from build123d import *

# Parameters (mm, degrees)
F1_DEPTH = 25
F2_R     = 2.5
F3_DEPTH = 15


with BuildPart() as f1:
    # F0 (on Front) → F1 (new body)
    with BuildSketch(Plane.XZ):
        Polygon((3.64, 10), (0, 0), (20, 0), (16.36, 10), (10, 10), align=None)
    extrude(amount=F1_DEPTH)

    # F2 (on Top) → F3 (join)
    with BuildSketch(Plane.XY):
        with Locations((10, -12.5)):
            Circle(F2_R)
    extrude(amount=F3_DEPTH)


solid = f1.part
Here's how the part is built. I have some questions about the finished solid (model axes, mm). A direction names the side the tool comes from. Give positions to 0.01 mm unless a question says otherwise; leave off trailing zeros. Order: outer loops, then holes, each group sorted by start corner. A loop starts at its lowest first (then second) coordinate and runs counter-clockwise, first axis right, second up. Notation, with made-up numbers: M -15,-3 L 29,-3 A22 ccw 29,9 Z; hole C -22,-11 d2. An arc over 180 degrees is marked long. Answer as a JSON object with one key per item and string values. Group by question number.
1) Suppose I cut it at B-B, the plane x = 10. Write out the boundary of the cut face in (y, z), plus the area to 3 significant figures.
2) Suppose I cut it at A-A, the plane y = -12.5. Write out the boundary of the cut face in (x, z), plus the area to 3 significant figures.
3) On a 3-axis mill with a long thin cutter (end or side, diameter ignored), from which of +Z, -Z, +X, -X, +Y, -Y can I reach the whole of each face in a straight line? I mean faces 1 (the flat face through (10, 0, 5)), 2 (the cylindrical face through (9.46, -14.94, 12.46)). Say none if no direction works.
4) Please list where these lines run through material, in increasing order: L1, parallel to Z at x = 7.5, y = -6; L2, parallel to Y at x = 11.25, z = 11.5; L3, parallel to X at y = -4.25, z = 6.75. Write a range as [from, to].
5) Suppose I cut it at C-C, the plane z = 12.5. Write out the boundary of the cut face in (x, y).
6) Suppose I cut it at D-D, the plane y = -5. Write out the boundary of the cut face in (x, z).
7) I'm going to push flat-ended pins straight in: pin 1 Ø1 at (y, z) = (-22, 4) entering from +X; pin 2 Ø5 at (y, z) = (-13.5, 4) entering from -X; pin 3 Ø4 at (x, z) = (4.5, 6) entering from +Y; pin 4 Ø6 at (y, z) = (-9, 2) entering from -X. Where does each tip first touch, or does it pass through?
Results found:
{
 "1": {"outline": "M -25,0 L 0,0 L 0,10 L -10,10 L -10,15 L -15,15 L -15,10 L -25,10 Z", "area": "275 mm²"},
 "2": {"outline": "M 0,0 L 20,0 L 16.36,10 L 12.5,10 L 12.5,15 L 7.5,15 L 7.5,10 L 3.64,10 Z", "area": "189 mm²"},
 "3": {"face 1": "+Z, -Z, +X, -X, +Y", "face 2": "+Z"},
 "4": {"L1": "[0, 10]", "L2": "[-14.67, -10.33]", "L3": "[2.46, 17.54]"},
 "5": {"outline": "C 10,-12.5 d5"},
 "6": {"outline": "M 0,0 L 20,0 L 16.36,10 L 3.64,10 Z"},
 "7": {"pin 1": "x = 18.73", "pin 2": "x = 0.55", "pin 3": "y = 0", "pin 4": "x = 0"}
}
